Geometry check sheet. Reference: the model listing, model coordinates, mm. A direction names the side the tool comes from. Round coordinates to 2 decimals unless told otherwise and drop trailing zeros. Order: outer loops, then holes, each group sorted by start corner. A loop starts at its lowest first (then second) coordinate and runs counter-clockwise, first axis right, second up.
(1) Gauge pin test, flat ends, axial feed: P1, Ø3, axis at x = 109, z = 273.5, coming from the +Y side; P2, Ø1.5, axis at x = 102, y = 12, coming from the -Z side; P3, Ø5, axis at y = 19, z = 55.5, coming from the +X side. Record the tip position at first contact, or that the pin passes through.
(2) Cross-section at B-B on y = 14.5. Enter the section's corners in (x, z) (3 decimals).
(3) Thickness scan on L1, parallel to X at y = 16.5, z = 146.5; L2, parallel to Y at x = 147.5, z = 69; L3, parallel to Z at x = 246, y = 6.25. Record the ranges inside material, lowest first.
(4) Set-up check for faces 1 (the face through (269.764, 10, 152)), 2 (the face through (125, 9, 0)), 3 (the face through (203.63, 20.62, 26.2)): record each of +Z, -Z, +X, -X, +Y, -Y from which the full face is reachable in a straight line by a thin tool's end or side.
(5) Cross-section at D-D on x = 139.5. Enter the section's corners in (y, z).
(6) Cross-section at A-A on z = 118. Enter the section's corners in (x, y), and give its area (3 significant figures).
(7) Draft check along X on faces 4 (the face through (155, 0, 150)), 5 (the face through (254.238, 9.658, 206.303)), 6 (the face through (279.756, 9.392, 259.728)), 7 (the face through (253.54, 9.66, 98.36)). Enter one of: pulls with the +X half, pulls with the -X half, needs draft (parallel to the pull), parting line crosses it, or undercut.
(8) Cross-section at C-C on z = 242. Enter the section's corners in (x, y) (3 decimals).
from build123d import *

# Parameters (mm, degrees)
BOSS_EXTRUDE1_DEPTH = 19.05
SKETCH4_R           = 25.488945224
SKETCH4_R_2         = 25.511029354
BOSS_EXTRUDE2_DEPTH = 3.175
CUT_EXTRUDE1_DEPTH  = 19.05


with BuildPart() as part:
    # Sketch3 → Boss-Extrude1 (new body)
    with BuildSketch(Plane(origin=(0, 0, 0), x_dir=(1, 0, 0), z_dir=(0, 1, 0))):
        Polygon((0, 0), (254, 0), (304.8, -88.9), (304.8, -215.9), (254, -304.8), (0, -304.8), align=None)
    extrude(amount=BOSS_EXTRUDE1_DEPTH)

    # Sketch4 → Boss-Extrude2 (add)
    with BuildSketch(Plane(origin=(0, 19.05, 0), x_dir=(1, 0, 0), z_dir=(0, 1, 0))):
        with Locations(Location((228.514370998, -31.725840718, 0), (0, 0, 270))):
            Circle(SKETCH4_R)
        with Locations(Location((228.514370998, -260.290019102, 0), (0, 0, 270))):
            Circle(SKETCH4_R_2)
    extrude(amount=BOSS_EXTRUDE2_DEPTH)

    # Sketch5 → Cut-Extrude1 (cut)
    with BuildSketch(Plane(origin=(0, 19.05, 0), x_dir=(1, 0, 0), z_dir=(0, 1, 0))):
        with BuildLine():
            Line((269.763997266, -114.231353373), (269.763997266, -190.431353373))
            ThreePointArc((269.763997266, -190.431353373), (253.888997266, -206.306353373), (238.013997266, -190.431353373))
            Line((238.013997266, -190.431353373), (238.013997266, -114.231353373))
            ThreePointArc((238.013997266, -114.231353373), (253.888997266, -98.356353373), (269.763997266, -114.231353373))
        make_face()
    extrude(amount=-CUT_EXTRUDE1_DEPTH, mode=Mode.SUBTRACT)


solid = part.part
Found:
1. P1: stops at y = 19.05
1. P2: stops at z = 0
1. P3: stops at x = 287.14
2. outline: (0, 0) - (254, 0) - (304.8, 88.9) - (304.8, 215.9) - (254, 304.8) - (0, 304.8) - close; hole (238.014, 114.231) arc R15.875 ccw to (269.764, 114.231) - (269.764, 190.431) arc R15.875 ccw to (238.014, 190.431) - close
3. L1: x = 0 to 238.01, 269.76 to 304.8
3. L2: y = 0 to 19.05
3. L3: z = 0 to 100.46, 204.21 to 304.8
4. face 1: +Y, -Y
4. face 2: -Z, +X, -X, +Y, -Y
4. face 3: +Y
5. outline: (0, 0) - (19.05, 0) - (19.05, 304.8) - (0, 304.8) - close
6. outline: (0, 0) - (238.01, 0) - (238.01, 19.05) - (0, 19.05) - close; (269.76, 0) - (304.8, 0) - (304.8, 19.05) - (269.76, 19.05) - close
6. area: 5,200 mm2
7. face 4: needs draft
7. face 5: undercut
7. face 6: pulls with the +X half
7. face 7: undercut
8. outline: (0, 0) - (289.886, 0) - (289.886, 19.05) - (246.299, 19.05) - (246.299, 22.225) - (210.73, 22.225) - (210.73, 19.05) - (0, 19.05) - close
